from build123d import *

# Parameters (mm, degrees)
CHAMFER1_SIZE       = 0.714375
EXTRUDE1_DEPTH      = 28.33544088
EXTRUDE1_DEPTH_BACK = 28.33544088
EXTRUDE3_DEPTH      = 28.335440933
EXTRUDE3_DEPTH_BACK = 28.335440933
SKETCH4_R           = 3.175
EXTRUDE4_DEPTH      = 14.2875
EXTRUDE6_DEPTH      = 28.335440933
EXTRUDE6_DEPTH_BACK = 28.335440933
SKETCH6_R           = 1.7859375


with BuildPart() as part:
    # Sketch1 → Revolve1 (revolve)
    with BuildSketch(Plane(origin=(0, 0, 0), x_dir=(1, 0, 0), z_dir=(0, 1, 0)), mode=Mode.PRIVATE) as revolve1_sk:
        Polygon((-25.4, 7.14375), (-11.043046875, 7.14375), (-11.043046875, 6.85403125), (-10.31875, 6.85403125), (-10.31875, 7.14375), (3.571875, 7.14375), (3.571875, 0), (-25.4, 0), align=None)
    revolve(revolve1_sk.sketch.rotate(Axis((-25.4, 0, 0), (1, 0, 0)), 180), axis=Axis((-25.4, 0, 0), (1, 0, 0)))

    # Chamfer1
    chamfer1_edges = [part.edges().sort_by_distance(p)[0] for p in [
        (-25.4, 0, -7.14375),
    ]]
    chamfer(chamfer1_edges, length=CHAMFER1_SIZE)

    # Sketch2 → Extrude1 (cut, two sides: drawn at the far end of the back side and taken through both)
    with BuildSketch(Plane(origin=(0, 0, 0), x_dir=(1, 0, 0), z_dir=(0, 1, 0)).offset(-EXTRUDE1_DEPTH_BACK)):
        with BuildLine():
            Line((-8.87015625, 7.14375), (7.14375, 7.14375))
            Line((7.14375, 7.14375), (7.14375, -7.14375))
            Line((7.14375, -7.14375), (-8.87015625, -7.14375))
            ThreePointArc((-8.87015625, -7.14375), (-7.823978284, -4.618052966), (-5.29828125, -3.571875))
            Line((-5.29828125, -3.571875), (0, -3.571875))
            ThreePointArc((0, -3.571875), (3.571875, 0), (0, 3.571875))
            Line((0, 3.571875), (-5.29828125, 3.571875))
            ThreePointArc((-5.29828125, 3.571875), (-7.823978284, 4.618052966), (-8.87015625, 7.14375))
        make_face()
    extrude(amount=EXTRUDE1_DEPTH + EXTRUDE1_DEPTH_BACK, mode=Mode.SUBTRACT)

    # Sketch3 → Extrude3 (cut, two sides: drawn at the far end of the back side and taken through both)
    with BuildSketch(Plane.XY.offset(-EXTRUDE3_DEPTH_BACK)):
        with BuildLine():
            Line((-7.08421875, 4.7577375), (7.14375, 4.7577375))
            Line((7.14375, 4.7577375), (7.14375, -4.7577375))
            Line((7.14375, -4.7577375), (-7.08421875, -4.7577375))
            ThreePointArc((-7.08421875, -4.7577375), (-8.87015625, 0), (-7.08421875, 4.7577375))
        make_face()
    extrude(amount=EXTRUDE3_DEPTH + EXTRUDE3_DEPTH_BACK, mode=Mode.SUBTRACT)

    # Sketch4 → Extrude4 (cut)
    with BuildSketch(Plane.ZY.offset(25.4)):
        Circle(SKETCH4_R)
    extrude(amount=-EXTRUDE4_DEPTH, mode=Mode.SUBTRACT)

    # Extrude5 cone 1 section (through the dimple's axis) → Extrude5 (revolve, cut)
    with BuildSketch(Plane(origin=(-11.1125, 0, 0), x_dir=(0, 0, 1), z_dir=(0, 1, 0))):
        Polygon((0, 0), (3.175, 0), (0, 3.175), align=None)
    revolve(axis=Axis((-11.1125, 0, 0), (1, 0, 0)), mode=Mode.SUBTRACT)

    # Sketch6 → Extrude6 (cut, two sides: drawn at the far end of the back side and taken through both)
    with BuildSketch(Plane(origin=(0, 0, 0), x_dir=(1, 0, 0), z_dir=(0, 1, 0)).offset(-EXTRUDE6_DEPTH_BACK)):
        with Locations(Location((0, 0, 0), (0, 0, 270))):
            Circle(SKETCH6_R)
    extrude(amount=EXTRUDE6_DEPTH + EXTRUDE6_DEPTH_BACK, mode=Mode.SUBTRACT)


solid = part.part
Work out the finished part from the listing and answer in its coordinate system (mm). A direction names the side the tool comes from. Give positions to 0.01 mm unless a question says otherwise; leave off trailing zeros. Loops run counter-clockwise (first coordinate to the right, second up) from the corner with the lowest first, then second, coordinate; pieces in that order, holes last. Notation, with made-up numbers: (9.25, 61) -> (32.25, 61) arc R18 ccw to (32.25, 70) -> close; hole circle Ø7 at (67, -15.75). An arc over 180 degrees is marked (long way). Use a Markdown table: item, result. Add a question column.
1. Find the intervals of material crossed by probe 1 along X at (y, z) = (-5.6, 0); probe 2 along Z at (x, y) = (0, -6.4); probe 3 along Y at (x, z) = (-4, -0.75), in increasing order.
2. Section A-A on x = -4 is taken. Determine the outline of the cut face in (y, z).
3. Section B-B on z = 0 is taken. State how many separate pieces and enclosed holes the cut face has, and give its area (3 significant figures).
4. For faces 1 (the flat face through (-3, -4.758, 0)), 2 (the cylindrical face through (-18.36, -3.1, -0.69)), 3 (the flat face through (-3, 5, -3.572)), determine the directions among +Z, -Z, +X, -X, +Y, -Y from which every point of the face is accessible in a straight line to the end or side of a thin tool.
5. Section C-C on x = -7.75 is taken. Determine the outline of the cut face in (y, z), and give its area (3 significant figures).
6. Determine the mould class of faces 4 (the cylindrical face through (-7.96, 3.77, -4.76)), 5 (the cylindrical face through (-10.68, 4.17, -5.44)), 6 (the flat face through (-3, 4.758, 0)) for opening direction X: released by +X, released by -X, zero draft, split by the parting line, or undercut.
7. Flat-ended cylindrical pins translate along their axes: pin 1 Ø7.5 at (y, z) = (0, 0) entering from +X; pin 2 Ø0.7 at (x, y) = (-2.5, -5.5) entering from +Z; pin 3 Ø0.7 at (x, y) = (-3.5, 6) entering from -Z; pin 4 Ø2 at (x, z) = (0, 0) entering from +Y. Find the tip coordinate at first contact, or state that the pin passes through.
Results below:
| question | item | result |
|---|---|---|
| 1 | probe 1 | x = -25.4 to -1.79, 1.79 to 3.57 |
| 1 | probe 2 | z = -3.17 to -1.79, 1.79 to 3.17 |
| 1 | probe 3 | y = -7.1 to -4.76, 4.76 to 7.1 |
| 2 | outline | (-6.19, -3.57) -> (-4.76, -3.57) -> (-4.76, 3.57) -> (-6.19, 3.57) arc R7.14 ccw to start; (4.76, -3.57) -> (6.19, -3.57) arc R7.14 ccw to (6.19, 3.57) -> (4.76, 3.57) -> close |
| 3 | separate pieces | 4 |
| 3 | enclosed holes | 0 |
| 3 | area | 183 mm^2 |
| 4 | face 1 | +Z, -Z, +X |
| 4 | face 2 | -X |
| 4 | face 3 | -Z, +X, +Y, -Y |
| 5 | outline | (-5.51, -4.55) -> (-3.87, -4.55) -> (-3.87, 4.55) -> (-5.51, 4.55) arc R7.14 ccw to start; (3.87, -4.55) -> (5.51, -4.55) arc R7.14 ccw to (5.51, 4.55) -> (3.87, 4.55) -> close |
| 5 | area | 50.2 mm^2 |
| 6 | face 4 | released by +X |
| 6 | face 5 | undercut |
| 6 | face 6 | zero draft |
| 7 | pin 1 | stops at x = -7.82 |
| 7 | pin 2 | stops at z = 3.57 |
| 7 | pin 3 | stops at z = -3.57 |
| 7 | pin 4 | passes through |
